The listing builds one solid part. Answer for the finished solid, in the listing's coordinates (mm). Round coordinates to 2 decimals unless told otherwise and drop trailing zeros. Write each loop counter-clockwise with the first axis right and the second up, starting at its lowest first coordinate (ties: lowest second). Pieces come first, ordered by that corner, then holes.
from build123d import *

# Parameters (mm, degrees)
SKETCH1_R              = 107.95
BOSS_EXTRUDE1_DEPTH    = 6.35
M3_CLEARANCE_HOLE1_D   = 3.2
CIRPATTERN1_COUNT      = 12
BOSS_EXTRUDE2_DEPTH    = 6.35
FILLET1_R              = 10
FILLET1_OF_MIRROR1_R   = 10
F_10_CLEARANCE_HOLE3_D = 4.9784
SKETCH11_R             = 5.1
CUT_EXTRUDE1_DEPTH     = 6.35


with BuildPart() as part:
    # Sketch1 → Boss-Extrude1 (new body)
    with BuildSketch(Plane(origin=(0, 0, 0), x_dir=(1, 0, 0), z_dir=(0, 1, 0))):
        with Locations(Location((0, 0, 0), (0, 0, 270))):
            Circle(SKETCH1_R)
    extrude(amount=BOSS_EXTRUDE1_DEPTH)

    # M3 Clearance Hole1 (through all)
    with Locations(Plane(origin=(0, 6.35, 0), x_dir=(1, 0, 0), z_dir=(0, 1, 0))):
        with Locations((0, 104.55)):
            m3_clearance_hole1 = Hole(M3_CLEARANCE_HOLE1_D / 2)

    # CirPattern1: M3 Clearance Hole1 ×12 about axis
    cirpattern1_axis = Axis((0, 0, 0), (0, 1, 0))
    for i in range(1, CIRPATTERN1_COUNT):
        add(m3_clearance_hole1.rotate(cirpattern1_axis, i * 360 / CIRPATTERN1_COUNT), mode=Mode.SUBTRACT)

    # Sketch2 → Boss-Extrude2 (add)
    with BuildSketch(Plane(origin=(0, 0, 0), x_dir=(1, 0, 0), z_dir=(0, 1, 0))):
        with BuildLine():
            Line((-156.234271247, 24.142135624), (-105.215777275, 24.142135624))
            ThreePointArc((-105.215777275, 24.142135624), (-107.95, 0), (-105.215777275, -24.142135624))
            Line((-105.215777275, -24.142135624), (-156.234271247, -24.142135624))
            Line((-156.234271247, -24.142135624), (-156.234271247, 24.142135624))
        make_face()
    boss_extrude2 = extrude(amount=BOSS_EXTRUDE2_DEPTH)

    # Fillet1
    fillet1_edges = [part.edges().sort_by_distance(p)[0] for p in [
        (-156.234271247, 3.175, -24.142135624),
        (-156.234271247, 3.175, 24.142135624),
        (-105.215777275, 3.175, 24.142135624),
        (-105.215777275, 3.175, -24.142135624),
    ]]
    fillet(fillet1_edges, radius=FILLET1_R)

    # Mirror1: Boss-Extrude2 across plane
    add(boss_extrude2.mirror(Plane(origin=(0, 0, 0), x_dir=(0, 0, 1), z_dir=(1, 0, 0))))

    # Fillet1 of Mirror1
    fillet1_of_mirror1_edges = [part.edges().sort_by_distance(p)[0] for p in [
        (156.234271247, 3.175, -24.142135624),
        (156.234271247, 3.175, 24.142135624),
        (105.215777275, 3.175, 24.142135624),
        (105.215777275, 3.175, -24.142135624),
    ]]
    fillet(fillet1_of_mirror1_edges, radius=FILLET1_OF_MIRROR1_R)

    # #10 Clearance Hole3 (through all)
    with Locations(Plane(origin=(0, 6.35, 0), x_dir=(1, 0, 0), z_dir=(0, 1, 0))):
        with Locations((-132.092135624, -14.142135624), (-117.95, 0), (-132.092135624, 14.142135624), (-146.234271247, 0), (146.234271247, 0), (132.092135624, 14.142135624), (117.95, 0), (132.092135624, -14.142135624)):
            Hole(F_10_CLEARANCE_HOLE3_D / 2)

    # Sketch11 → Cut-Extrude1 (cut)
    with BuildSketch(Plane(origin=(0, 6.35, 0), x_dir=(1, 0, 0), z_dir=(0, 1, 0))):
        with Locations(Location((-66.262216278, 42.831398459, 0), (0, 0, 270))):
            Circle(SKETCH11_R)
        with Locations(Location((-77.461022456, 15, 0), (0, 0, 270))):
            Circle(SKETCH11_R)
        with Locations(Location((-77.461022456, -15, 0), (0, 0, 270))):
            Circle(SKETCH11_R)
        with Locations(Location((-66.262216278, -42.831398459, 0), (0, 0, 270))):
            Circle(SKETCH11_R)
        with Locations(Location((0, 25.519524251, 0), (0, 0, 270))):
            Circle(SKETCH11_R)
        with Locations(Location((-24.270509831, 7.885966682, 0), (0, 0, 270))):
            Circle(SKETCH11_R)
        with Locations(Location((24.270509831, 7.885966682, 0), (0, 0, 270))):
            Circle(SKETCH11_R)
        with Locations(Location((-15, -20.645728807, 0), (0, 0, 270))):
            Circle(SKETCH11_R)
        with Locations(Location((15, -20.645728807, 0), (0, 0, 270))):
            Circle(SKETCH11_R)
        with Locations(Location((-55.980762114, -15, 0), (0, 0, 270))):
            Circle(SKETCH11_R)
        with Locations(Location((-40.980762114, -40.980762114, 0), (0, 0, 270))):
            Circle(SKETCH11_R)
        with Locations(Location((-15, -55.980762114, 0), (0, 0, 270))):
            Circle(SKETCH11_R)
        with Locations(Location((15, -55.980762114, 0), (0, 0, 270))):
            Circle(SKETCH11_R)
        with Locations(Location((-55.980762114, 15, 0), (0, 0, 270))):
            Circle(SKETCH11_R)
        with Locations(Location((55.980762114, -15, 0), (0, 0, 270))):
            Circle(SKETCH11_R)
        with Locations(Location((40.980762114, -40.980762114, 0), (0, 0, 270))):
            Circle(SKETCH11_R)
        with Locations(Location((66.262216278, -42.831398459, 0), (0, 0, 270))):
            Circle(SKETCH11_R)
        with Locations(Location((77.461022456, -15, 0), (0, 0, 270))):
            Circle(SKETCH11_R)
        with Locations(Location((77.461022456, 15, 0), (0, 0, 270))):
            Circle(SKETCH11_R)
        with Locations(Location((66.262216278, 42.831398459, 0), (0, 0, 270))):
            Circle(SKETCH11_R)
        with Locations(Location((55.980762114, 15, 0), (0, 0, 270))):
            Circle(SKETCH11_R)
        with Locations(Location((40.980762114, 40.980762114, 0), (0, 0, 270))):
            Circle(SKETCH11_R)
        with Locations(Location((15, 55.980762114, 0), (0, 0, 270))):
            Circle(SKETCH11_R)
        with Locations(Location((-15, 55.980762114, 0), (0, 0, 270))):
            Circle(SKETCH11_R)
        with Locations(Location((-40.980762114, 40.980762114, 0), (0, 0, 270))):
            Circle(SKETCH11_R)
    extrude(amount=-CUT_EXTRUDE1_DEPTH, mode=Mode.SUBTRACT)


solid = part.part
1. For a pull along Z with two mould halves and no side action, classify faces 1 (the face through (129, 3, 24.142)), 2 (the face through (10.475, 3.219, -53.627)), 3 (the face through (130, 3, -24.142)) as released by +Z, released by -Z, zero draft, split by the parting line, or undercut.
Geometry says:
face 1: released by +Z
face 2: undercut
face 3: released by -Z
2. Section C-C on x = -98 is taken. Determine the outline of the cut face in (y, z), plus the area to 3 significant figures.
Geometry says:
outline: (0, -45.27) - (6.35, -45.27) - (6.35, 45.27) - (0, 45.27) - close
area: 575 mm2
3. Given pin 1 (3 mm diameter, centred on x = -52.27, z = -90.54, fed in from +Y), flat-ended and moving along its own axis, determine where the tip first touches the part or whether it passes through.
Geometry says:
pin 1: passes through
4. Section B-B on y = 3.5 is taken. Give the number of separate pieces and of enclosed holes in the cut face, plus the area to 3 significant figures.
Geometry says:
separate pieces: 1
enclosed holes: 45
area: 39,000 mm2
5. Section A-A on x = -15 is taken. Determine the outline of the cut face in (y, z).
Geometry says:
outline: (0, -106.9) - (6.35, -106.9) - (6.35, -61.08) - (0, -61.08) - close; (0, -50.88) - (6.35, -50.88) - (6.35, 15.55) - (0, 15.55) - close; (0, 25.75) - (6.35, 25.75) - (6.35, 50.88) - (0, 50.88) - close; (0, 61.08) - (6.35, 61.08) - (6.35, 106.9) - (0, 106.9) - close
6. Straight lines are drawn through the part: line 1 along X through (y, z) = (3.25, -56.5); line 2 along X through (y, z) = (5.75, 37); line 3 along Z through (x, y) = (117.95, 2.5). For each, find the intervals that lie inside material, in ascending order.
Geometry says:
line 1: x = -91.98 to -20.07, -9.93 to 9.93, 20.07 to 91.98
line 2: x = -101.41 to -44.17, -37.79 to 37.79, 44.17 to 101.41
line 3: z = -24.14 to -2.49, 2.49 to 24.14
